from build123d import *

# Parameters (mm, degrees)
SKETCH_1_W               = 20
SKETCH_1_H               = 20
SKETCH_1_R               = 2
SKETCH_1_R_2             = 2.15
EXTRUDE_1_DEPTH          = 345
CUT_EXTRUDE_1_REACH      = 347.29
PATTERN_CIRCULAR_1_COUNT = 4
FILLET_1_R               = 0.3
CUT_EXTRUDE_2_DEPTH      = 346.289733412
CUT_EXTRUDE_2_DEPTH_BACK = 346.289733412
SKETCH_2_R               = 2.5
SKETCH_4_R               = 2.15
CUT_EXTRUDE_3_DEPTH      = 346.723878361
SKETCH_6_R               = 2.15
SKETCH_6_R_2             = 1.97965
CUT_EXTRUDE_4_DEPTH      = 346.723878361
SKETCH_7_W               = 20
SKETCH_7_H               = 116.62
CUT_EXTRUDE_5_DEPTH      = 346.723878361


with BuildPart() as part:
    # Sketch 1 → Extrude 1 (new body)
    with BuildSketch(Plane.XY):
        Rectangle(SKETCH_1_W, SKETCH_1_H)
        with Locations((-7, 7)):
            Circle(SKETCH_1_R, mode=Mode.SUBTRACT)
        with Locations((-7, -7)):
            Circle(SKETCH_1_R, mode=Mode.SUBTRACT)
        Circle(SKETCH_1_R_2, mode=Mode.SUBTRACT)
        with Locations((7, 7)):
            Circle(SKETCH_1_R, mode=Mode.SUBTRACT)
        with Locations((7, -7)):
            Circle(SKETCH_1_R, mode=Mode.SUBTRACT)
    extrude(amount=EXTRUDE_1_DEPTH)

    # Sketch 1_3 → Cut-Extrude 1 (cut, up to next)
    with BuildSketch(Plane.XY, mode=Mode.PRIVATE) as cut_extrude_1_sk1:
        with BuildLine():
            Line((-8.5, 2.65), (-10, 2.65))
            Line((-10, 2.65), (-10, -2.65))
            Line((-10, -2.65), (-8.5, -2.65))
            Line((-8.5, -2.65), (-8.5, -4.15))
            Line((-8.5, -4.15), (-4.503166667, -4.15))
            ThreePointArc((-4.503166667, -4.15), (-3.3, 0), (-4.503166667, 4.15))
            Line((-4.503166667, 4.15), (-8.5, 4.15))
            Line((-8.5, 4.15), (-8.5, 2.65))
        make_face()
    cut_extrude_1_tool1 = extrude(cut_extrude_1_sk1.sketch, amount=CUT_EXTRUDE_1_REACH, mode=Mode.PRIVATE) & part.part
    cut_extrude_1 = cut_extrude_1_tool1.solids().sort_by_distance((-6.606913, 0, 0))[0]
    add(cut_extrude_1, mode=Mode.SUBTRACT)

    # Pattern Circular 1: Cut-Extrude 1 ×4 about axis
    pattern_circular_1_axis = Axis((0, 0, 0), (0, 0, 1))
    for i in range(1, PATTERN_CIRCULAR_1_COUNT):
        add(cut_extrude_1.rotate(pattern_circular_1_axis, i * 360 / PATTERN_CIRCULAR_1_COUNT), mode=Mode.SUBTRACT)

    # Fillet 1
    fillet_1_edges = [part.edges().sort_by_distance(p)[0] for p in [
        (-10, -10, 172.5),
        (10, -10, 172.5),
        (10, 10, 172.5),
        (-10, 10, 172.5),
    ]]
    fillet(fillet_1_edges, radius=FILLET_1_R)

    # Sketch 2 → Cut-Extrude 2 (cut, two sides: drawn at the far end of the back side and taken through both)
    with BuildSketch(Plane(origin=(0, 0, 0), x_dir=(0, 0, -1), z_dir=(1, 0, 0)).offset(-CUT_EXTRUDE_2_DEPTH_BACK)):
        with Locations((-25, 0)):
            Circle(SKETCH_2_R)
    extrude(amount=CUT_EXTRUDE_2_DEPTH + CUT_EXTRUDE_2_DEPTH_BACK, mode=Mode.SUBTRACT)

    # Sketch 4 → Cut-Extrude 3 (cut, through all)
    with BuildSketch(Plane(origin=(0, 10, 0), x_dir=(1, 0, 0), z_dir=(0, 1, 0))):
        with Locations(Location((0, -303, 0), (0, 0, 270))):
            Circle(SKETCH_4_R)
    extrude(amount=-CUT_EXTRUDE_3_DEPTH, mode=Mode.SUBTRACT)

    # Sketch 6 → Cut-Extrude 4 (cut, through all)
    with BuildSketch(Plane(origin=(0, 10, 0), x_dir=(1, 0, 0), z_dir=(0, 1, 0))):
        with Locations(Location((0, -236.9, 0), (0, 0, 270))):
            Circle(SKETCH_6_R)
        with Locations(Location((0, -184.9, 0), (0, 0, 270))):
            Circle(SKETCH_6_R)
        with Locations(Location((0, -10.15, 0), (0, 0, 270))):
            Circle(SKETCH_6_R_2)
        with Locations(Location((0, -62.15, 0), (0, 0, 270))):
            Circle(SKETCH_6_R)
    extrude(amount=-CUT_EXTRUDE_4_DEPTH, mode=Mode.SUBTRACT)

    # Sketch 7 → Cut-Extrude 5 (cut, through all)
    with BuildSketch(Plane(origin=(0, 10, 0), x_dir=(1, 0, 0), z_dir=(0, 1, 0))):
        with Locations((0, -58.31)):
            Rectangle(SKETCH_7_W, SKETCH_7_H)
    extrude(amount=-CUT_EXTRUDE_5_DEPTH, mode=Mode.SUBTRACT)


solid = part.part
Could you check a few things on this model? Use its own coordinates, in mm. A direction names the side the tool comes from. Give positions to 0.01 mm unless a question says otherwise; leave off trailing zeros.
1. For faces 4 (the flat face through (-6, 4.15, 229)), 5 (the flat face through (6, 10, 229)), which set-ups out of +Z, -Z, +X, -X, +Y, -Y let a thin tool reach every point of the face, with its end or its side?
2. We'd pull the mould along X, two halves only. Please class faces 1 (the flat face through (6, -10, 229)), 2 (the cylindrical face through (-3.3, -0.1, 229.2)), 3 (the flat face through (-10, -6, 229)): pulls with the +X half, pulls with the -X half, needs draft (parallel to the pull), parting line crosses it, or undercut.
3. Suppose I cut it at A-A (x = 0). Give the number of separate pieces and of enclosed holes in the cut face, plus the area to 3 significant figures.
4. I need wall thicknesses on L1, parallel to X at y = -7, z = 260; L2, parallel to Z at x = 0, y = -2.5. Which ranges of each line are inside material? Lowest first, please.
Solved:
1. face 4: +Z, -Z
1. face 5: +Z, -Z, +X, -X, +Y
2. face 1: needs draft
2. face 2: undercut
2. face 3: pulls with the -X half
3. separate pieces: 8
3. enclosed holes: 0
3. area: 496 mm2
4. L1: x = -10 to -9, -5 to -4.15, 4.15 to 5, 9 to 10
4. L2: z = 116.62 to 182.75, 187.05 to 234.75, 239.05 to 300.85, 305.15 to 345
